Verification items for the finished model (mm, model axes). Round coordinates to 2 decimals unless told otherwise and drop trailing zeros. Write each loop counter-clockwise with the first axis right and the second up, starting at its lowest first coordinate (ties: lowest second). Pieces come first, ordered by that corner, then holes.
Autodesk Inventor part; units mm, degrees
ref_plane "CP_XY" through (0, 0, 0) normal (1, 0, 0) x (0, 0, -1)
ref_plane "CP_YZ" through (0, 0, 0) normal (0, 0, -1) x (0, 1, 0)
ref_plane "CP_ZX" through (0, 0, 0) normal (0, 1, 0) x (1, 0, 0)
sketch "Sketch_1" plane through (0, 0, 0) normal (0, 0, 1) x (1, 0, 0)
  line L0 (0, 0) -> (-9.5, 0)
  line L1 (-9.5, 0) -> (-9.5, 2.0095)
  line L2 (-9.5, 2.0095) -> (-9.0095, 2.5)
  line L3 (-9.0095, 2.5) -> (-0.75, 2.5)
  line L4 (-0.75, 2.5) -> (0, 1.75)
  line L5 (0, 1.75) -> (0, 0)
  line L6 (0, 0) -> (-9.5, 0)
revolve "Revolution1" add sketch "Sketch_1" angle 360 about axis through (0, 0, 0) along (1, 0, 0)
thread "Thread1"
sketch "Sketch_2" plane through (-9.5, 0, 0) normal (-1, 0, 0) x (0, 1, 0)
  line L0 (-1.25, 0.7217) -> (-1.25, -0.7217)
  line L1 (-1.25, -0.7217) -> (0, -1.4434)
  line L2 (0, -1.4434) -> (1.25, -0.7217)
  line L3 (1.25, -0.7217) -> (1.25, 0.7217)
  line L4 (1.25, 0.7217) -> (0, 1.4434)
  line L5 (0, 1.4434) -> (-1.25, 0.7217)
extrude "Extrusion1" cut sketch "Sketch_2" against normal blind 2
sketch "Sketch_3" plane through (0, 0, 0) normal (0, 0, 1) x (1, 0, 0)
  line L0 (-6.7783, 0) -> (-7.5, 0)
  line L1 (-7.5, 0) -> (-7.5, 1.25)
  line L2 (-7.5, 1.25) -> (-6.7783, 0)
  line L3 (-6.7783, 0) -> (-7.5, 0)
revolve "Revolution2" cut sketch "Sketch_3" angle 360 about axis through (-6.7783, 0, 0) along (1, 0, 0)
ref_plane "CP_XY" through (0, 0, 0) normal (1, 0, 0) x (0, 0, -1)
ref_plane "CP_YZ" through (0, 0, 0) normal (0, 0, -1) x (0, 1, 0)
ref_plane "CP_ZX" through (0, 0, 0) normal (0, 1, 0) x (1, 0, 0)
properties part number "SET-SCREW5-9.5"
Q1. Material ranges on line 1 along Y through (x, z) = (-8, 0.4); line 2 along Y through (x, z) = (-7.5, 1.8); line 3 along Z through (x, y) = (-0.5, 0.6), recorded low to high.
Recorded:
line 1: y = -2.47 to -1.25, 1.25 to 2.47
line 2: y = -1.73 to 1.73
line 3: z = -2.17 to 2.17
Q2. Sectioned sample at A-A (x = -5.75). Enter the section's corners in (y, z), plus the area to 3 significant figures.
Recorded:
outline: circle Ø5 at (0, 0)
area: 19.6 mm2
Q3. Release check for a two-part mould opening along Y. For faces 1 (the flat face through (0, 0, 0)), 2 (the cylindrical face through (-4.82, -0.54, -2.44)), 3 (the flat face through (-8.514, 0.616, 1.088)) record: released by +Y, released by -Y, zero draft, split by the parting line, or undercut.
Recorded:
face 1: zero draft
face 2: split by the parting line
face 3: undercut
